Design review of the part shown in the three views and the two pictorial views. Dimensions are in mm from the part's minimum x, y and z. Round coordinates to 2 decimals unless told otherwise and drop trailing zeros. Loops run counter-clockwise (first coordinate to the right, second up) from the corner with the lowest first, then second, coordinate; pieces in that order, holes last. Notation, with made-up numbers: M 53,85 L 77,85 A17 ccw 77,115 Z; hole C 87.25,11 d11. An arc over 180 degrees is marked long. One line per question, with ' | ' between items. Start each with the question number.
1) We need section B-B (y = 736.6). Give the boundary of the cut face in (x, z), and give its area (3 significant figures).
2) For pin 1 Ø12 at (x, y) = (506, 261.5) entering from +Z; pin 2 Ø6 at (y, z) = (759, 89) entering from -X; pin 3 Ø1.5 at (y, z) = (759, 95) entering from -X (1 decimal), all flat-tipped, find the tip position at first contact; note any pin that passes through.
3) We need section D-D (y = 132). Give the boundary of the cut face in (x, z) (1 decimal), and give its area (3 significant figures).
4) We need section A-A (z = 256.5). Give the boundary of the cut face in (x, y), and give its area (3 significant figures).
5) Mouldability with a two-part tool opening along Y and no side actions: class the marked faces 1 and 2 as pulls with the +Y half, pulls with the -Y half, needs draft (parallel to the pull), parting line crosses it, or undercut.
6) For probe 1 along Z at (x, y) = (692.5, 713); probe 2 along X at (y, z) = (171, 377) (1 decimal); probe 3 along X at (y, z) = (736.5, 342), list the stretches that pass through material, from the lowest coordinate up. Write a range as from..to.
7) We need section C-C (x = 1142). Give the boundary of the cut face in (y, z).
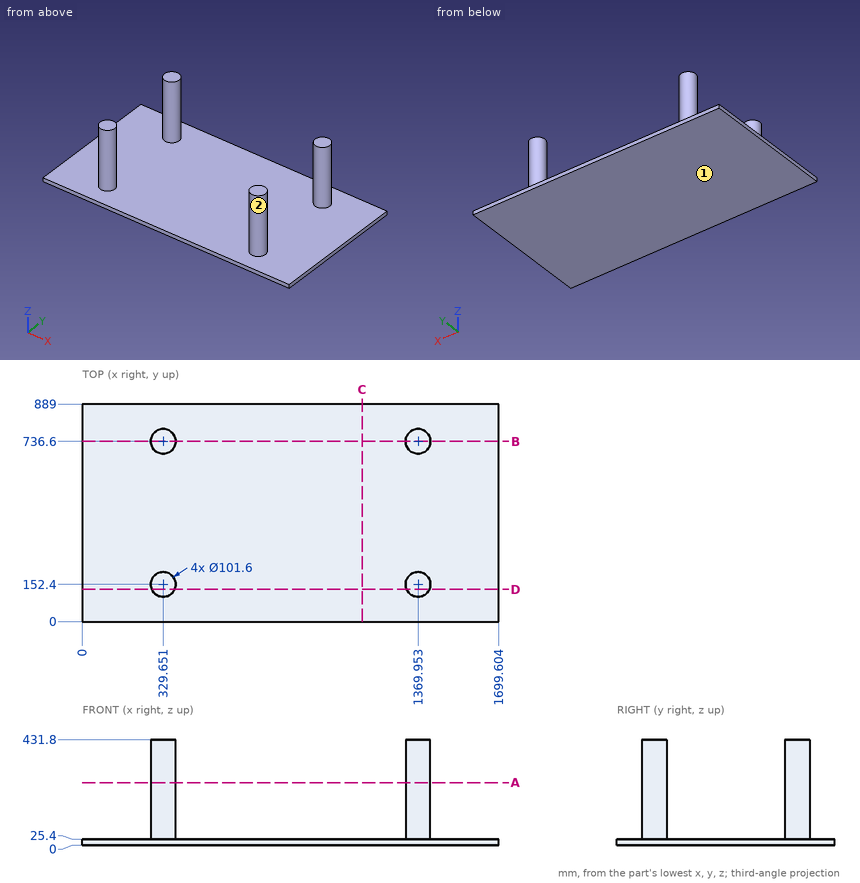
Answers below:
1) outline: M 0,0 L 1699.6,0 L 1699.6,25.4 L 1420.75,25.4 L 1420.75,431.8 L 1319.15,431.8 L 1319.15,25.4 L 380.45,25.4 L 380.45,431.8 L 278.85,431.8 L 278.85,25.4 L 0,25.4 Z | area: 126,000 mm^2
2) pin 1: z = 25.4 | pin 2: x = 282.7 | pin 3: x = 283.7
3) outline: M 0,0 L 1699.6,0 L 1699.6,25.4 L 1416.5,25.4 L 1416.5,431.8 L 1323.4,431.8 L 1323.4,25.4 L 376.2,25.4 L 376.2,431.8 L 283.1,431.8 L 283.1,25.4 L 0,25.4 Z | area: 119,000 mm^2
4) outline: C 329.65,152.4 d101.6; C 329.65,736.6 d101.6; C 1369.95,152.4 d101.6; C 1369.95,736.6 d101.6 | area: 32,400 mm^2
5) face 1: needs draft | face 2: undercut
6) probe 1: 0..25.4 | probe 2: 282.4..376.9, 1322.7..1417.2 | probe 3: 278.85..380.45, 1319.15..1420.75
7) outline: M 0,0 L 889,0 L 889,25.4 L 0,25.4 Z
